Source: CAD feature listing. Evaluate the final solid. Frame: model axes, mm. Face numbers are marked on the shaded views. Give positions to 0.01 mm unless a question says otherwise; leave off trailing zeros. Loops run counter-clockwise (first coordinate to the right, second up) from the corner with the lowest first, then second, coordinate; pieces in that order, holes last.
from build123d import *

# Parameters (mm, degrees)
SKETCH1_W            = 74
SKETCH1_H            = 30
BOSS_EXTRUDE1_DEPTH  = 5
M6_CLEARANCE_HOLE1_D = 6.6
SKETCH5_R            = 1.4
CUT_EXTRUDE1_DEPTH   = 5
SKETCH6_R            = 1.4
CUT_EXTRUDE2_DEPTH   = 5
CHAMFER1_SIZE        = 0.5


with BuildPart() as part:
    # Sketch1 → Boss-Extrude1 (new body)
    with BuildSketch(Plane.XY):
        with Locations((37, 15)):
            Rectangle(SKETCH1_W, SKETCH1_H)
    extrude(amount=BOSS_EXTRUDE1_DEPTH)

    # M6 Clearance Hole1 (through all)
    with Locations(Plane.XY.offset(5)):
        with Locations((17, 6.5), (57, 6.5)):
            Hole(M6_CLEARANCE_HOLE1_D / 2)

    # Sketch5 → Cut-Extrude1 (cut)
    with BuildSketch(Plane.XY.offset(5)):
        with Locations((59, 22.5)):
            Circle(SKETCH5_R)
        with Locations((59, 14.5)):
            Circle(SKETCH5_R)
    extrude(amount=-CUT_EXTRUDE1_DEPTH, mode=Mode.SUBTRACT)

    # Sketch6 → Cut-Extrude2 (cut)
    with BuildSketch(Plane.XY.offset(5)):
        with Locations((5, 20)):
            Circle(SKETCH6_R)
        with Locations((13, 20)):
            Circle(SKETCH6_R)
    extrude(amount=-CUT_EXTRUDE2_DEPTH, mode=Mode.SUBTRACT)

    # Chamfer1
    chamfer1_edges = [part.edges().sort_by_distance(p)[0] for p in [
        (74, 15, 5),
        (37, 30, 5),
        (60.3, 6.5, 5),
        (60.3, 6.5, 0),
        (20.3, 6.5, 5),
        (20.3, 6.5, 0),
        (0, 15, 5),
        (37, 30, 0),
        (74, 15, 0),
        (37, 0, 0),
        (0, 15, 0),
        (57.6, 22.5, 0),
        (57.6, 22.5, 5),
        (37, 0, 5),
        (57.6, 14.5, 0),
        (57.6, 14.5, 5),
        (0, 30, 2.5),
        (74, 30, 2.5),
        (74, 0, 2.5),
        (0, 0, 2.5),
        (3.6, 20, 0),
        (3.6, 20, 5),
        (11.6, 20, 0),
        (11.6, 20, 5),
    ]]
    chamfer(chamfer1_edges, length=CHAMFER1_SIZE)


solid = part.part
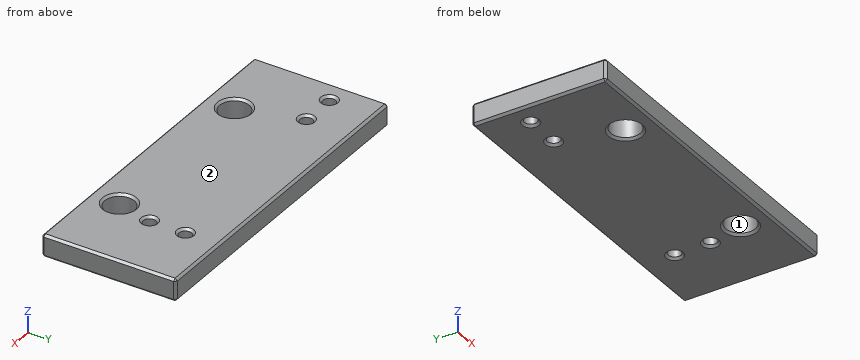
1) Pull-direction query (Y, two-part tool) for the marked faces 1 and 2; classes: released by +Y, released by -Y, zero draft, split by the parting line, or undercut.
Checks:
face 1: undercut
face 2: zero draft
2) Cut plane D-D (y = 6.5). Return loops of the section in (x, z).
Checks:
outline: (0, 0.5) - (0.5, 0) - (13.2, 0) - (13.7, 0.5) - (13.7, 4.5) - (13.2, 5) - (0.5, 5) - (0, 4.5) - close; (20.3, 0.5) - (20.8, 0) - (53.2, 0) - (53.7, 0.5) - (53.7, 4.5) - (53.2, 5) - (20.8, 5) - (20.3, 4.5) - close; (60.3, 0.5) - (60.8, 0) - (73.5, 0) - (74, 0.5) - (74, 4.5) - (73.5, 5) - (60.8, 5) - (60.3, 4.5) - close
3) Cut plane B-B (z = 3.35). Return loops of the section in (x, y), and give its area (3 significant figures).
Checks:
outline: (0, 0.5) - (0.5, 0) - (73.5, 0) - (74, 0.5) - (74, 29.5) - (73.5, 30) - (0.5, 30) - (0, 29.5) - close; hole circle Ø2.8 at (5, 20); hole circle Ø2.8 at (13, 20); hole circle Ø6.6 at (17, 6.5); hole circle Ø6.6 at (57, 6.5); hole circle Ø2.8 at (59, 14.5); hole circle Ø2.8 at (59, 22.5)
area: 2,130 mm2
4) Cut plane C-C (y = 14.5). Return loops of the section in (x, z).
Checks:
outline: (0, 0.5) - (0.5, 0) - (57.1, 0) - (57.6, 0.5) - (57.6, 4.5) - (57.1, 5) - (0.5, 5) - (0, 4.5) - close; (60.4, 0.5) - (60.9, 0) - (73.5, 0) - (74, 0.5) - (74, 4.5) - (73.5, 5) - (60.9, 5) - (60.4, 4.5) - close
5) Contact query for a flat-ended pin moving along its axis: P1, Ø3.5, axis at x = 5, y = 20, coming from the +Z side. Output: stop coordinate, or through.
Checks:
P1: stops at z = 4.85
6) Cut plane A-A (x = 17). Return loops of the section in (y, z), and give its area (3 significant figures).
Checks:
outline: (0, 0.5) - (0.5, 0) - (2.7, 0) - (3.2, 0.5) - (3.2, 4.5) - (2.7, 5) - (0.5, 5) - (0, 4.5) - close; (9.8, 0.5) - (10.3, 0) - (29.5, 0) - (30, 0.5) - (30, 4.5) - (29.5, 5) - (10.3, 5) - (9.8, 4.5) - close
area: 116 mm2
7) Ray query, probe 1 along Y at (x, z) = (5, 2.5); probe 2 along X at (y, z) = (9.5, 2.25); probe 3 along Y at (x, z) = (17, 1). Return the intervals inside material, ascending.
Checks:
probe 1: y = 0 to 18.6, 21.4 to 30
probe 2: x = 0 to 15.63, 18.37 to 55.63, 58.37 to 74
probe 3: y = 0 to 3.2, 9.8 to 30
